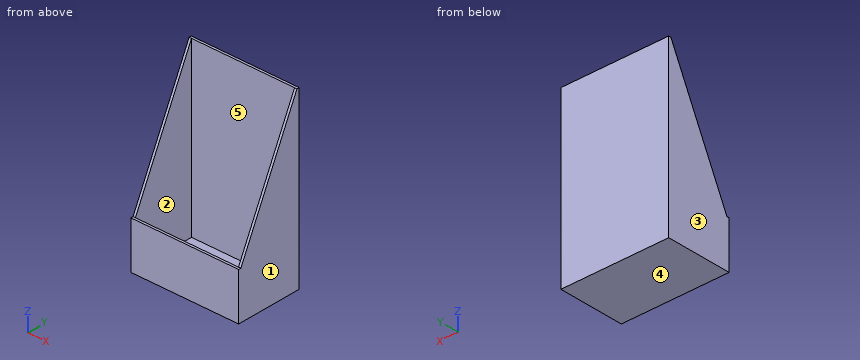
```python
from build123d import *

# Parameters (mm, degrees)
F0_W     = 114
F0_H     = 70
F1_DEPTH = 185
F5_DEPTH = 114
F3_W     = 109
F3_H     = 65
F6_DEPTH = 182.501


with BuildPart() as f1:
    # F0 (on Top) → F1 (new body)
    with BuildSketch(Plane.XY):
        with Locations((-57, -35)):
            Rectangle(F0_W, F0_H)
    extrude(amount=F1_DEPTH)

    # F4 (on Right) → F5 (cut, through all)
    with BuildSketch(Plane.YZ):
        Polygon((-70, 185), (-70, 50), (-67.5, 50), (-2.5, 185), align=None)
    extrude(amount=-F5_DEPTH, mode=Mode.SUBTRACT)

    # F3 (on offset) → F6 (cut, through all)
    with BuildSketch(Plane.XY.offset(2.5)):
        with Locations((-57, -35)):
            Rectangle(F3_W, F3_H)
    extrude(amount=F6_DEPTH, mode=Mode.SUBTRACT)


solid = f1.part
```
Can you work these out from the model? Positions are in its coordinate system, mm. Face numbers are marked on the shaded views. A direction names the side the tool comes from. Coordinates: 2 decimals unless noted, no trailing zeros. Loops run counter-clockwise (first coordinate to the right, second up) from the corner with the lowest first, then second, coordinate; pieces in that order, holes last. Notation, with made-up numbers: (22, 65) -> (45, 65) arc R15 cw to (45, 87) -> close; hole circle Ø4 at (-11, 6). An arc over 180 degrees is marked (long way). Answer as a JSON object with one key per item and string values.
1) Imagine slicing it at C-C (z = 99.5). Please give me the cut outline in (x, y), then the cut area to 3 significant figures.
Results:
{"outline": "(-114, -43.67) -> (-111.5, -43.67) -> (-111.5, -2.5) -> (-2.5, -2.5) -> (-2.5, -43.67) -> (0, -43.67) -> (0, 0) -> (-114, 0) -> close", "area": "491 mm^2"}
2) Thinking about a two-plate mould opening in X: for the marked faces 3, 4 and 5, which applies, pulls with the +X half, pulls with the -X half, needs draft (parallel to the pull), parting line crosses it, or undercut?
Results:
{"face 3": "pulls with the -X half", "face 4": "needs draft", "face 5": "undercut"}
3) Imagine slicing it at A-A (z = 37.5). Please give me the cut outline in (x, y).
Results:
{"outline": "(-114, -70) -> (0, -70) -> (0, 0) -> (-114, 0) -> close; hole (-111.5, -67.5) -> (-2.5, -67.5) -> (-2.5, -2.5) -> (-111.5, -2.5) -> close"}
4) Imagine slicing it at B-B (x = -87). Please give me the cut outline in (y, z), then the cut area to 3 significant figures.
Results:
{"outline": "(-70, 0) -> (0, 0) -> (0, 185) -> (-2.5, 185) -> (-2.5, 2.5) -> (-67.5, 2.5) -> (-67.5, 50) -> (-70, 50) -> close", "area": "750 mm^2"}
5) If I drill on line 1 (X direction, y = -41, z = 57); line 2 (Y direction, x = -104.5, z = 46); line 3 (Z direction, x = -88, y = -19.5), over which ranges is the centre line in solid material (lowest first)?
Results:
{"line 1": "x = -114 to -111.5, -2.5 to 0", "line 2": "y = -70 to -67.5, -2.5 to 0", "line 3": "z = 0 to 2.5"}
6) For P1, Ø2, axis at x = -36, y = -69.5, coming from the +Z side; P2, Ø5, axis at x = -44.5, z = 152.5, coming from the -Y side; P3, Ø4, axis at x = -80, y = -20, coming from the -Z side; P4, Ø19.5, axis at x = -62, y = -45, coming from the +Z side, each with a flat end and sliding along its axis, tell me the tip position at first contact or that it passes through.
Results:
{"P1": "stops at z = 50", "P2": "stops at y = -2.5", "P3": "stops at z = 0", "P4": "stops at z = 2.5"}
7) For the marked faces 1 and 2, which set-ups out of +Z, -Z, +X, -X, +Y, -Y let a thin tool reach every point of the face, with its end or its side?
Results:
{"face 1": "+Z, -Z, +X, +Y, -Y", "face 2": "+Z"}
